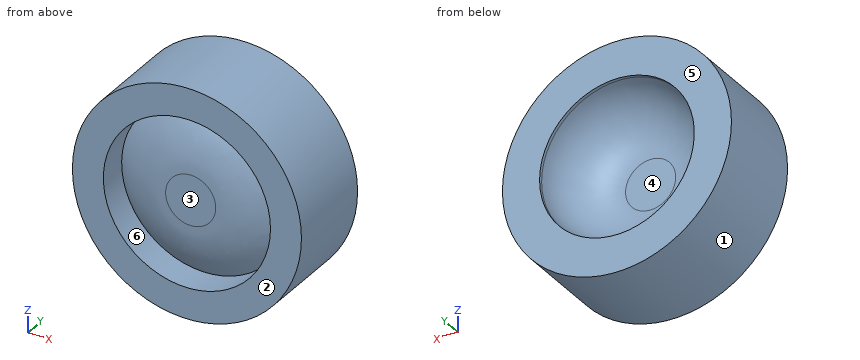
from build123d import *

# Parameters (mm, degrees)
F0_R     = 9.398
F1_DEPTH = 7.62
F2_T     = -3.048
F3_R     = 4.2924717139
F4_T     = -2.54


with BuildPart() as f1:
    # F0 (on Front) → F1 (new body)
    with BuildSketch(Plane.XZ):
        with Locations((3.7124650553, 24.0670088679)):
            Circle(F0_R)
    extrude(amount=F1_DEPTH)

    # F2
    f2_openings = [f1.faces().sort_by_distance(p)[0] for p in [
        (3.712465, 0, 24.067009),
    ]]
    offset(amount=F2_T, openings=f2_openings)

    # F3
    f3_edges = [f1.edges().sort_by_distance(p)[0] for p in [
        (-2.637535, -4.572, 24.067009),
    ]]
    fillet(f3_edges, radius=F3_R)

    # F4
    f4_openings = [f1.faces().sort_by_distance(p)[0] for p in [
        (3.712465, -7.62, 24.067009),
    ]]
    offset(amount=F4_T, openings=f4_openings)


solid = f1.part
Model file for the job. Use its own axes, mm. Face numbers are marked on the shaded views. A direction names the side the tool comes from. Coordinates: 2 decimals unless noted, no trailing zeros. Return JSON: item names as keys, results as strings. Group by question number.
Item 1: Pull direction X, two halves, no side cores. Call the marked faces 1, 2 and 3: pulls with the +X half, pulls with the -X half, needs draft (parallel to the pull), parting line crosses it, or undercut.
Item 2: Flat gauge pins, fed straight in: P1, Ø10, axis at x = 3.71, z = 24.07, coming from the +Y side; P2, Ø1.5, axis at x = 7, y = -2.5, coming from the +Z side; P3, Ø3.5, axis at x = 4, z = 25, coming from the -Y side. Where does each tip first touch, or does it go through?
Item 3: Wall check: line 1 along Z through (x, y) = (4.25, -6.5); line 2 along Z through (x, y) = (1, -2.75); line 3 along Z through (x, y) = (10, -6.5). Give the ranges that are in metal, low to high. Write a range as [from, to].
Item 4: Tool access for the marked faces 4, 5 and 6: list every direction of +Z, -Z, +X, -X, +Y, -Y with a clear straight run to the whole face (end or side of a thin tool).
Item 5: Saw through at A-A on y = -5.5. State how many separate pieces and enclosed holes the cut face has, then the cut area to 3 significant figures.
Values found:
{
 "1": {"face 1": "parting line crosses it", "face 2": "needs draft", "face 3": "undercut"},
 "2": {"P1": "stops at y = -3.4", "P2": "stops at z = 33.12", "P3": "stops at y = -7.11"},
 "3": {"line 1": "z = [14.68, 17.23], [19.21, 28.92], [30.9, 33.45]", "line 2": "z = [15.07, 19.2], [28.93, 33.07]", "line 3": "z = [17.08, 21.33], [26.81, 31.05]"},
 "4": {"face 4": "+Y", "face 5": "+Z, -Z, +X, -X, +Y", "face 6": "-Y"},
 "5": {"separate pieces": "2", "enclosed holes": "1", "area": "261 mm2"}
}
